Could you check a few things on this drawing? It's one solid part, dimensions in mm from its lowest x, y, z. A direction names the side the tool comes from. Give positions to 0.01 mm unless a question says otherwise; leave off trailing zeros. Loops run counter-clockwise (first coordinate to the right, second up) from the corner with the lowest first, then second, coordinate; pieces in that order, holes last. Notation, with made-up numbers: (79.25, 15.5) - (97.25, 15.5) arc R27 cw to (97.25, 53.5) - close; hole circle Ø8 at (-7.75, 57). An arc over 180 degrees is marked (long way). Use a Markdown table: item, result.
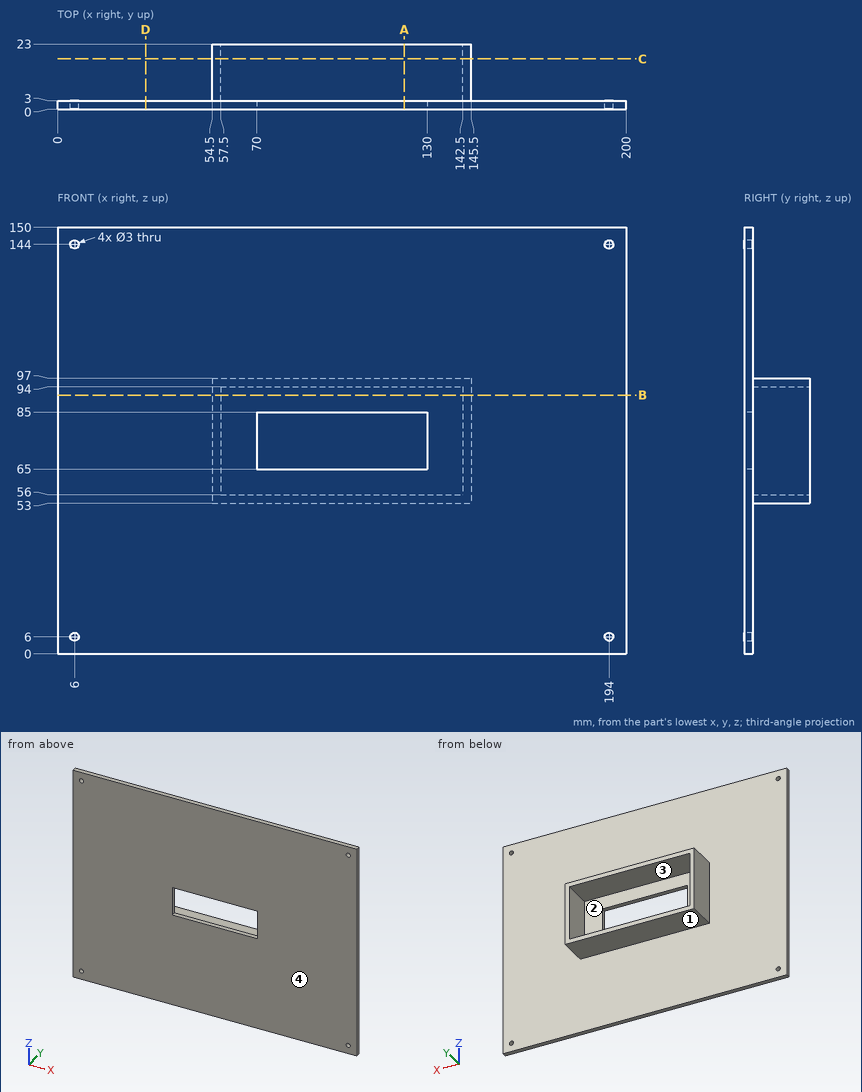
(1) Suppose I cut it at C-C on y = 17.75. Write out the boundary of the cut face in (x, z).
A:
| item | result |
|---|---|
| outline | (54.5, 53) - (145.5, 53) - (145.5, 97) - (54.5, 97) - close; hole (57.5, 56) - (142.5, 56) - (142.5, 94) - (57.5, 94) - close |
(2) On a 3-axis mill with a long thin cutter (end or side, diameter ignored), from which of +Z, -Z, +X, -X, +Y, -Y can I reach the whole of each face in a straight line? I mean the marked faces 1 and 2. Say none if no direction works.
A:
| item | result |
|---|---|
| face 1 | -Z, +X, -X, +Y |
| face 2 | +Y |
(3) We'd pull the mould along X, two halves only. Please class the marked faces 3 and 4: pulls with the +X half, pulls with the -X half, needs draft (parallel to the pull), parting line crosses it, or undercut.
A:
| item | result |
|---|---|
| face 3 | undercut |
| face 4 | needs draft |
(4) If I drill on line 1 (X direction, y = 1.4, z = 144); line 2 (Z direction, x = 6, y = 1); line 3 (Z direction, x = 104, y = 8.75), over which ranges is the centre line in solid material (lowest first)?
A:
| item | result |
|---|---|
| line 1 | 0 to 4.5, 7.5 to 192.5, 195.5 to 200 |
| line 2 | 0 to 4.5, 7.5 to 142.5, 145.5 to 150 |
| line 3 | 53 to 56, 94 to 97 |
(5) Suppose I cut it at B-B on z = 91. Write out the boundary of the cut face in (x, y).
A:
| item | result |
|---|---|
| outline | (0, 0) - (200, 0) - (200, 3) - (145.5, 3) - (145.5, 23) - (142.5, 23) - (142.5, 3) - (57.5, 3) - (57.5, 23) - (54.5, 23) - (54.5, 3) - (0, 3) - close |
(6) Will these pins go through, and if not, where does the flat tip stop? pin 1 (6 mm diameter, centred on y = 11, z = 77, fed in from +X); pin 2 (1.5 mm diameter, centred on y = 1.5, z = 77.5, fed in from -X); pin 3 (4 mm diameter, centred on x = 63, y = 11, fed in from -Z).
A:
| item | result |
|---|---|
| pin 1 | x = 145.5 |
| pin 2 | x = 0 |
| pin 3 | z = 53 |
(7) Suppose I cut it at D-D on x = 31. Write out the boundary of the cut face in (y, z), plus the area to 3 significant figures.
A:
| item | result |
|---|---|
| outline | (0, 0) - (3, 0) - (3, 150) - (0, 150) - close |
| area | 450 mm2 |
(8) Suppose I cut it at A-A on x = 122. Write out the boundary of the cut face in (y, z).
A:
| item | result |
|---|---|
| outline | (0, 0) - (3, 0) - (3, 53) - (23, 53) - (23, 56) - (3, 56) - (3, 65) - (0, 65) - close; (0, 85) - (3, 85) - (3, 94) - (23, 94) - (23, 97) - (3, 97) - (3, 150) - (0, 150) - close |
